Read the model definition and answer for the solid it produces. Units are mm, in the model's axes. A direction names the side the tool comes from. Give positions to 0.01 mm unless a question says otherwise; leave off trailing zeros. Write each loop counter-clockwise with the first axis right and the second up, starting at its lowest first coordinate (ties: lowest second). Pieces come first, ordered by that corner, then holes. Notation, with made-up numbers: (48, 28.25) -> (93, 28.25) arc R15 ccw to (93, 53.25) -> close; hole circle Ø5 at (38, 86). An arc over 180 degrees is marked (long way). Answer as CSV lines item,"result". Start each with the question number.
1. For a pull along Z with two mould halves and no side action, classify faces 5 (the flat face through (0.547, 634.609, -418.795)), 6 (the flat face through (501, 622, 25.4)), 7 (the flat face through (116.63, 634.61, -401.08)) as pulls with the +Z half, pulls with the -Z half, needs draft (parallel to the pull), parting line crosses it, or undercut.
2. The part is cut by section A-A, the plane y = 498. Determine the outline of the cut face in (x, z), and give its area (3 significant figures).
3. The part is cut by section D-D, the plane x = 833. Determine the outline of the cut face in (y, z), and give its area (3 significant figures).
4. Given pin 1 (4 mm diameter, centred on x = 603.5, z = -452, fed in from -Y); pin 2 (15 mm diameter, centred on y = 260.5, z = -535, fed in from -X); pin 3 (15 mm diameter, centred on y = 403.5, z = -524.5, fed in from +X), each flat-ended and moving along its own axis, determine where each tip first touches the part or whether it passes through.
5. Find the intervals of material crossed by line 1 (Z direction, x = 23, y = 477.5); line 2 (X direction, y = 31, z = -512.5); line 3 (Y direction, x = 515, z = -317), in increasing order.
6. The part is cut by section B-B, the plane x = 567. Determine the outline of the cut face in (y, z).
7. A tool of negligible diameter and unlimited length cuts with its end or side. For faces 1 (the flat face through (965.2, 301, -25)), 2 (the flat face through (25, 301, -558.8)), 3 (the flat face through (190.946, 634.609, -489.798)), 4 (the flat face through (990, 301, 0)), from which of +Z, -Z, +X, -X, +Y, -Y can it reach the whole face along a straight path? Write none if from no direction.
8. The part is cut by section C-C, the plane z = -527.5. Determine the outline of the cut face in (x, y).
from build123d import *

# Parameters (mm, degrees)
SKETCH1_W             = 50.8
SKETCH1_H             = 50.8
BOSS_EXTRUDE1_DEPTH   = 609.6
BOSS_EXTRUDE1_2_DEPTH = 609.6
BOSS_EXTRUDE1_3_DEPTH = 609.6
BOSS_EXTRUDE1_4_DEPTH = 609.6
SKETCH2_W             = 1066.8
SKETCH2_H             = 609.6
BOSS_EXTRUDE2_DEPTH   = 25.4
SKETCH3_W             = 203.2
SKETCH3_H             = 114.3
SKETCH3_W_2           = 431.8
SKETCH3_H_2           = 127
CUT_EXTRUDE1_DEPTH    = 0.79375


with BuildPart() as part:
    # Sketch1 → Boss-Extrude1 (new body)
    with BuildSketch(Plane(origin=(0, 0, 0), x_dir=(1, 0, 0), z_dir=(0, 1, 0))):
        with Locations((25.4, 25.4)):
            Rectangle(SKETCH1_W, SKETCH1_H)
    extrude(amount=BOSS_EXTRUDE1_DEPTH)



with BuildPart() as body_2:
    # Sketch1 → Boss-Extrude1 2 (new body)
    with BuildSketch(Plane(origin=(0, 0, 0), x_dir=(1, 0, 0), z_dir=(0, 1, 0))):
        with Locations((25.4, 533.4)):
            Rectangle(SKETCH1_W, SKETCH1_H)
    extrude(amount=BOSS_EXTRUDE1_2_DEPTH)


with BuildPart() as body_3:
    # Sketch1 → Boss-Extrude1 3 (new body)
    with BuildSketch(Plane(origin=(0, 0, 0), x_dir=(1, 0, 0), z_dir=(0, 1, 0))):
        with Locations((990.6, 533.4)):
            Rectangle(SKETCH1_W, SKETCH1_H)
    extrude(amount=BOSS_EXTRUDE1_3_DEPTH)


with BuildPart() as body_4:
    # Sketch1 → Boss-Extrude1 4 (new body)
    with BuildSketch(Plane(origin=(0, 0, 0), x_dir=(1, 0, 0), z_dir=(0, 1, 0))):
        with Locations((990.6, 25.4)):
            Rectangle(SKETCH1_W, SKETCH1_H)
    extrude(amount=BOSS_EXTRUDE1_4_DEPTH)


with BuildPart() as part_1:
    add(part.part)

    add(body_2.part)  # Boss-Extrude2 merges body 2

    add(body_3.part)  # Boss-Extrude2 merges body 3

    add(body_4.part)  # Boss-Extrude2 merges body 4
    # Sketch2 → Boss-Extrude2 (add)
    with BuildSketch(Plane(origin=(0, 609.6, 0), x_dir=(1, 0, 0), z_dir=(0, 1, 0))):
        with Locations((508, 279.4)):
            Rectangle(SKETCH2_W, SKETCH2_H)
    extrude(amount=BOSS_EXTRUDE2_DEPTH)

    # Sketch3 → Cut-Extrude1 (cut)
    with BuildSketch(Plane(origin=(0, 635, 0), x_dir=(1, 0, 0), z_dir=(0, 1, 0))):
        Polygon((210.765672654, 435.342380006), (19.82013211, 365.843886882), (-19.272770272, 473.250753438), (171.672770272, 542.749246562), align=None)
        with Locations((508, 501.65)):
            Rectangle(SKETCH3_W, SKETCH3_H)
        Polygon((844.327229728, 542.749246562), (1035.272770272, 473.250753438), (996.17986789, 365.843886882), (805.234327346, 435.342380006), align=None)
        with Locations((508, 96.68413443)):
            Rectangle(SKETCH3_W_2, SKETCH3_H_2)
    extrude(amount=-CUT_EXTRUDE1_DEPTH, mode=Mode.SUBTRACT)


solid = part_1.part
Results found:
1,face 5,"undercut"
1,face 6,"pulls with the +Z half"
1,face 7,"undercut"
2,outline,"(0, -558.8) -> (50.8, -558.8) -> (50.8, -508) -> (0, -508) -> close; (0, -50.8) -> (50.8, -50.8) -> (50.8, 0) -> (0, 0) -> close; (965.2, -558.8) -> (1016, -558.8) -> (1016, -508) -> (965.2, -508) -> close; (965.2, -50.8) -> (1016, -50.8) -> (1016, 0) -> (965.2, 0) -> close"
2,area,"10,300 mm²"
3,outline,"(609.6, -584.2) -> (635, -584.2) -> (635, -511.63) -> (634.21, -511.63) -> (634.21, -425.24) -> (635, -425.24) -> (635, 25.4) -> (609.6, 25.4) -> close"
3,area,"15,400 mm²"
4,pin 1,"stops at y = 609.6"
4,pin 2,"stops at x = 0"
4,pin 3,"stops at x = 1016"
5,line 1,"z = -558.8 to -508, -50.8 to 0"
5,line 2,"x = 0 to 50.8, 965.2 to 1016"
5,line 3,"y = 609.6 to 635"
6,outline,"(609.6, -584.2) -> (635, -584.2) -> (635, -558.8) -> (634.21, -558.8) -> (634.21, -444.5) -> (635, -444.5) -> (635, -160.18) -> (634.21, -160.18) -> (634.21, -33.18) -> (635, -33.18) -> (635, 25.4) -> (609.6, 25.4) -> close"
7,face 1,"+Z, -Z, -Y"
7,face 2,"-Z, +X, -X, -Y"
7,face 3,"+Y"
7,face 4,"+Z, +X, -X, -Y"
8,outline,"(-25.4, 609.6) -> (0, 609.6) -> (0, 0) -> (50.8, 0) -> (50.8, 609.6) -> (965.2, 609.6) -> (965.2, 0) -> (1016, 0) -> (1016, 609.6) -> (1041.4, 609.6) -> (1041.4, 635) -> (886.22, 635) -> (886.22, 634.21) -> (838.78, 634.21) -> (838.78, 635) -> (609.6, 635) -> (609.6, 634.21) -> (406.4, 634.21) -> (406.4, 635) -> (177.22, 635) -> (177.22, 634.21) -> (129.78, 634.21) -> (129.78, 635) -> (-25.4, 635) -> close"
